```python
from build123d import *

# Parameters (mm, degrees)
EXTRUDE_1_DEPTH  = 7.8
EXTRUDE_3_DEPTH  = 1.2
SKETCH_9_4_R     = 8.191420507
EXTRUDE_4_DEPTH  = 4
SKETCH_9_5_R     = 1.750016101
EXTRUDE_5_DEPTH  = 3
EXTRUDE_7_DEPTH  = 1
EXTRUDE_8_DEPTH  = 1
EXTRUDE_9_DEPTH  = 1
SKETCH_11_R      = 1.061990405
EXTRUDE_10_DEPTH = 0.08


with BuildPart() as part:
    # 草图1 → 凸台-拉伸1 (new body)
    with BuildSketch(Plane.XY):
        with BuildLine():
            Line((26.75, -80.45), (-26.75, -80.45))
            ThreePointArc((-26.75, -80.45), (-35.235281374, -76.935281374), (-38.75, -68.45))
            Line((-38.75, -68.45), (-38.75, 68.45))
            ThreePointArc((-38.75, 68.45), (-35.235281374, 76.935281374), (-26.75, 80.45))
            Line((-26.75, 80.45), (26.75, 80.45))
            ThreePointArc((26.75, 80.45), (35.235281374, 76.935281374), (38.75, 68.45))
            Line((38.75, 68.45), (38.75, -68.45))
            ThreePointArc((38.75, -68.45), (35.235281374, -76.935281374), (26.75, -80.45))
        make_face()
    extrude(amount=EXTRUDE_1_DEPTH)

    # 草图9 → 凸台-拉伸3 (add)
    with BuildSketch(Plane(origin=(0, 0, 0), x_dir=(-1, 0, 0), z_dir=(0, 0, -1))):
        with BuildLine():
            Line((-27.75, 75.45), (-5.75, 75.45))
            ThreePointArc((-5.75, 75.45), (-0.093145751, 73.106854249), (2.25, 67.45))
            Line((2.25, 67.45), (2.25, 45.45))
            ThreePointArc((2.25, 45.45), (-0.093145751, 39.793145751), (-5.75, 37.45))
            Line((-5.75, 37.45), (-27.75, 37.45))
            ThreePointArc((-27.75, 37.45), (-33.406854249, 39.793145751), (-35.75, 45.45))
            Line((-35.75, 45.45), (-35.75, 67.45))
            ThreePointArc((-35.75, 67.45), (-33.406854249, 73.106854249), (-27.75, 75.45))
        make_face()
    extrude(amount=EXTRUDE_3_DEPTH)

    # 草图9<4> → 凸台-拉伸4 (add)
    with BuildSketch(Plane(origin=(0, 0, 0), x_dir=(-1, 0, 0), z_dir=(0, 0, -1))):
        with Locations((-25.75, 65.45)):
            Circle(SKETCH_9_4_R)
        with Locations((-7.75, 57.360656258)):
            Circle(SKETCH_9_4_R)
        with Locations((-25.75, 47.45)):
            Circle(SKETCH_9_4_R)
    extrude(amount=EXTRUDE_4_DEPTH)

    # 草图9<5> → 凸台-拉伸5 (add)
    with BuildSketch(Plane(origin=(0, 0, 0), x_dir=(-1, 0, 0), z_dir=(0, 0, -1))):
        with Locations((-9.360421126, 69.360656258)):
            Circle(SKETCH_9_5_R)
    extrude(amount=EXTRUDE_5_DEPTH)

    # 草图12 → 凸台-拉伸7 (add)
    with BuildSketch(Plane.ZY.offset(38.75)):
        with BuildLine():
            Line((4.686466023, 51.699871834), (4.686466023, 46.158543385))
            ThreePointArc((4.686466023, 46.158543385), (3.550247732, 45.022325093), (2.41402944, 46.158543385))
            Line((2.41402944, 46.158543385), (2.41402944, 51.699871834))
            ThreePointArc((2.41402944, 51.699871834), (3.550247732, 52.836090125), (4.686466023, 51.699871834))
        make_face()
    extrude(amount=EXTRUDE_7_DEPTH)

    # 草图12<3> → 凸台-拉伸8 (add)
    with BuildSketch(Plane.ZY.offset(38.75)):
        with BuildLine():
            Line((4.686466023, 51.699871834), (4.686466023, 46.158543385))
            ThreePointArc((4.686466023, 46.158543385), (3.550247732, 45.022325093), (2.41402944, 46.158543385))
            Line((2.41402944, 46.158543385), (2.41402944, 51.699871834))
            ThreePointArc((2.41402944, 51.699871834), (3.550247732, 52.836090125), (4.686466023, 51.699871834))
        make_face()
        with BuildLine():
            Line((2.585183967, 27.92697733), (2.585183967, 39.027618957))
            ThreePointArc((2.585183967, 39.027618957), (3.550247732, 39.992682722), (4.515311496, 39.027618957))
            Line((4.515311496, 39.027618957), (4.515311496, 27.92697733))
            ThreePointArc((4.515311496, 27.92697733), (3.550247732, 26.961913565), (2.585183967, 27.92697733))
        make_face()
        with BuildLine():
            Line((2.34585079, 8.760131584), (2.34585079, 22.388503734))
            ThreePointArc((2.34585079, 22.388503734), (3.550247732, 23.592900676), (4.754644674, 22.388503734))
            Line((4.754644674, 22.388503734), (4.754644674, 8.760131584))
            ThreePointArc((4.754644674, 8.760131584), (3.550247732, 7.555734642), (2.34585079, 8.760131584))
        make_face()
    extrude(amount=EXTRUDE_8_DEPTH)

    # 草图13 → 凸台-拉伸9 (add)
    with BuildSketch(Plane(origin=(38.75, 0, 0), x_dir=(0, 0, -1), z_dir=(1, 0, 0))):
        with BuildLine():
            Line((-3.041514771, 35.957715301), (-3.041514771, 18.606690775))
            ThreePointArc((-3.041514771, 18.606690775), (-4.183029543, 17.465176003), (-5.324544314, 18.606690775))
            Line((-5.324544314, 18.606690775), (-5.324544314, 35.957715301))
            ThreePointArc((-5.324544314, 35.957715301), (-4.183029543, 37.099230072), (-3.041514771, 35.957715301))
        make_face()
    extrude(amount=EXTRUDE_9_DEPTH)

    # 草图11 → 凸台-拉伸10 (add)
    with BuildSketch(Plane(origin=(0, 0, -1.2), x_dir=(-1, 0, 0), z_dir=(0, 0, -1))):
        with Locations((-9.68745595, 42.936842594)):
            Circle(SKETCH_11_R)
    extrude(amount=EXTRUDE_10_DEPTH)


solid = part.part
```
Check sheet for the modelled part. Datum: model origin and axes. Units: mm. A direction names the side the tool comes from. Round coordinates to 2 decimals unless told otherwise and drop trailing zeros. Write each loop counter-clockwise with the first axis right and the second up, starting at its lowest first coordinate (ties: lowest second). Pieces come first, ordered by that corner, then holes. Notation, with made-up numbers: M -26.75,80 L -11.75,80 A8 ccw -11.75,84 Z; hole C -11,5 d3. An arc over 180 degrees is marked long. Write item = value, one per line. Start each with the question number.
1. Scan lines: line 1 (Y direction, x = 28.5, z = -0.25); line 2 (Z direction, x = 2, y = 37); line 3 (Z direction, x = 0, y = 52). Record each from-to range of solid material in increasing order. Write a range as [from, to].
2. Release check for a two-part mould opening along X. For faces 1 (the flat face through (0, 80.45, 4)), 2 (the flat face through (38.75, 1, 4)), 3 (the flat face through (16.5, 56.7, -1.2)) record: pulls with the +X half, pulls with the -X half, needs draft (parallel to the pull), parting line crosses it, or undercut.
3. Section check A-A, the plane y = -27. Record the cut outline in (x, z).
4. Tool access check on faces 4 (the cylindrical face through (9.588, 71.096, -2.087)), 5 (the cylindrical face through (0.031, 39.856, -0.592)), 6 (the cylindrical face through (33.469, 73.044, -0.592)), 7 (the cylindrical face through (0.156, 73.169, -0.592)). Record the directions out of +Z, -Z, +X, -X, +Y, -Y that give a thin tool (end or side, any length) a straight path to the whole face; none if there is none.
5. Gauge pin test, flat ends, axial feed: pin 1 (1 mm diameter, centred on x = 10.5, z = -2.5, fed in from -Y); pin 2 (4 mm diameter, centred on y = 40.5, z = -2.5, fed in from +X); pin 3 (5 mm diameter, centred on x = -28.5, y = 33.5, fed in from -Z). Record the tip position at first contact, or that the pin passes through.
Results found:
q1.line_1 = [37.49, 75.41]
q1.line_2 = [0, 7.8]
q1.line_3 = [-1.2, 7.8]
q2.face_1 = needs draft
q2.face_2 = pulls with the +X half
q2.face_3 = undercut
q3.outline = M -38.75,0 L 38.75,0 L 38.75,7.8 L -38.75,7.8 Z
q4.face_4 = -Z
q4.face_5 = -Z, -X, -Y
q4.face_6 = -Z, +X, +Y
q4.face_7 = -Z, -X, +Y
q5.pin_1 = 49.48
q5.pin_2 = 34.98
q5.pin_3 = 0
